Can you work these out from the model? Positions are in its coordinate system, mm. A direction names the side the tool comes from. Coordinates: 2 decimals unless noted, no trailing zeros. Order: outer loops, then holes, each group sorted by start corner. A loop starts at its lowest first (then second) coordinate and runs counter-clockwise, first axis right, second up.
```python
from build123d import *

# Parameters (mm, degrees)
SKETCH2_R           = 6
SKETCH2_R_2         = 1.5
BOSS_EXTRUDE1_DEPTH = 1.15
SKETCH3_R           = 4.4
BOSS_EXTRUDE2_DEPTH = 3.2
SKETCH4_R           = 0.75
BOSS_EXTRUDE3_DEPTH = 1.15
CIRPATTERN1_COUNT   = 2
CUT_EXTRUDE1_DEPTH  = 10


with BuildPart() as part:
    # Sketch2 → Boss-Extrude1 (new, symmetric)
    with BuildSketch(Plane(origin=(0, 0, 0), x_dir=(1, 0, 0), z_dir=(0, 1, 0))):
        with Locations(Location((0, 0, 0), (0, 0, 270))):
            Circle(SKETCH2_R)
        with Locations(Location((0, 0, 0), (0, 0, 270))):
            Circle(SKETCH2_R_2, mode=Mode.SUBTRACT)
    extrude(amount=BOSS_EXTRUDE1_DEPTH, both=True)

    # Sketch3 → Boss-Extrude2 (add)
    with BuildSketch(Plane(origin=(0, 1.15, 0), x_dir=(1, 0, 0), z_dir=(0, 1, 0))):
        with Locations(Location((0, 0, 0), (0, 0, 270))):
            Circle(SKETCH3_R)
        with BuildLine():
            Line((0.107421435, 2.898009771), (0.338399731, 2.678709694))
            Line((0.338399731, 2.678709694), (0.61665913, 2.83367809))
            ThreePointArc((0.61665913, 2.83367809), (0.721200673, 2.808891167), (0.824752316, 2.780248841))
            Line((0.824752316, 2.780248841), (0.993936292, 2.510396512))
            Line((0.993936292, 2.510396512), (1.301992734, 2.591295993))
            ThreePointArc((1.301992734, 2.591295993), (1.397085655, 2.541289372), (1.490260976, 2.48779465))
            Line((1.490260976, 2.48779465), (1.587020181, 2.184345885))
            Line((1.587020181, 2.184345885), (1.905517346, 2.186093238))
            ThreePointArc((1.905517346, 2.186093238), (1.985186607, 2.11400902), (2.062131058, 2.039023173))
            Line((2.062131058, 2.039023173), (2.080385755, 1.721044772))
            Line((2.080385755, 1.721044772), (2.389311295, 1.643530205))
            ThreePointArc((2.389311295, 1.643530205), (2.448550984, 1.553897705), (2.504429862, 1.46213237))
            Line((2.504429862, 1.46213237), (2.443033042, 1.149604087))
            Line((2.443033042, 1.149604087), (2.722976028, 0.997698125))
            ThreePointArc((2.722976028, 0.997698125), (2.758063897, 0.896149284), (2.789366126, 0.793370413))
            Line((2.789366126, 0.793370413), (2.652175577, 0.505929549))
            Line((2.652175577, 0.505929549), (2.885546163, 0.289177003))
            ThreePointArc((2.885546163, 0.289177003), (2.894277512, 0.182092507), (2.899036259, 0.074758075))
            Line((2.899036259, 0.074758075), (2.694672167, -0.169534403))
            Line((2.694672167, -0.169534403), (2.866806821, -0.437514174))
            ThreePointArc((2.866806821, -0.437514174), (2.848633027, -0.543405812), (2.826549281, -0.648551587))
            Line((2.826549281, -0.648551587), (2.567852594, -0.834345885))
            Line((2.567852594, -0.834345885), (2.667935462, -1.136714727))
            ThreePointArc((2.667935462, -1.136714727), (2.623998452, -1.234759946), (2.576459817, -1.331110368))
            Line((2.576459817, -1.331110368), (2.279685399, -1.446732346))
            Line((2.279685399, -1.446732346), (2.301427906, -1.764491312))
            ThreePointArc((2.301427906, -1.764491312), (2.234488404, -1.84852957), (2.164481907, -1.930030589))
            Line((2.164481907, -1.930030589), (1.848277186, -1.968215294))
            Line((1.848277186, -1.968215294), (1.790313171, -2.281398419))
            ThreePointArc((1.790313171, -2.281398419), (1.704577232, -2.346149284), (1.616501638, -2.40767989))
            Line((1.616501638, -2.40767989), (1.30073492, -2.366028036))
            Line((1.30073492, -2.366028036), (1.166706475, -2.654956874))
            ThreePointArc((1.166706475, -2.654956874), (1.067561203, -2.696351809), (0.966950626, -2.734045809))
            Line((0.966950626, -2.734045809), (0.671462695, -2.615174535))
            Line((0.671462695, -2.615174535), (0.469791321, -2.861694623))
            ThreePointArc((0.469791321, -2.861694623), (0.363466377, -2.877132634), (0.25664255, -2.888621575))
            Line((0.25664255, -2.888621575), (0, -2.7))
            Line((0, -2.7), (-0.25664255, -2.888621575))
            ThreePointArc((-0.25664255, -2.888621575), (-0.363466377, -2.877132634), (-0.469791321, -2.861694623))
            Line((-0.469791321, -2.861694623), (-0.671462695, -2.615174535))
            Line((-0.671462695, -2.615174535), (-0.966950626, -2.734045809))
            ThreePointArc((-0.966950626, -2.734045809), (-1.067561203, -2.696351809), (-1.166706475, -2.654956874))
            Line((-1.166706475, -2.654956874), (-1.30073492, -2.366028036))
            Line((-1.30073492, -2.366028036), (-1.616501638, -2.40767989))
            ThreePointArc((-1.616501638, -2.40767989), (-1.704577232, -2.346149284), (-1.790313171, -2.281398419))
            Line((-1.790313171, -2.281398419), (-1.848277186, -1.968215294))
            Line((-1.848277186, -1.968215294), (-2.164481907, -1.930030589))
            ThreePointArc((-2.164481907, -1.930030589), (-2.234488404, -1.84852957), (-2.301427906, -1.764491312))
            Line((-2.301427906, -1.764491312), (-2.279685399, -1.446732346))
            Line((-2.279685399, -1.446732346), (-2.576459817, -1.331110368))
            ThreePointArc((-2.576459817, -1.331110368), (-2.623998452, -1.234759946), (-2.667935462, -1.136714727))
            Line((-2.667935462, -1.136714727), (-2.567852594, -0.834345885))
            Line((-2.567852594, -0.834345885), (-2.826549281, -0.648551587))
            ThreePointArc((-2.826549281, -0.648551587), (-2.848633027, -0.543405812), (-2.866806821, -0.437514174))
            Line((-2.866806821, -0.437514174), (-2.694672167, -0.169534403))
            Line((-2.694672167, -0.169534403), (-2.899036259, 0.074758075))
            ThreePointArc((-2.899036259, 0.074758075), (-2.894277512, 0.182092507), (-2.885546163, 0.289177003))
            Line((-2.885546163, 0.289177003), (-2.652175577, 0.505929549))
            Line((-2.652175577, 0.505929549), (-2.789366126, 0.793370413))
            ThreePointArc((-2.789366126, 0.793370413), (-2.758063897, 0.896149284), (-2.722976028, 0.997698125))
            Line((-2.722976028, 0.997698125), (-2.443033042, 1.149604087))
            Line((-2.443033042, 1.149604087), (-2.504429862, 1.46213237))
            ThreePointArc((-2.504429862, 1.46213237), (-2.448550984, 1.553897705), (-2.389311295, 1.643530205))
            Line((-2.389311295, 1.643530205), (-2.080385755, 1.721044772))
            Line((-2.080385755, 1.721044772), (-2.062131058, 2.039023173))
            ThreePointArc((-2.062131058, 2.039023173), (-1.985186607, 2.11400902), (-1.905517346, 2.186093238))
            Line((-1.905517346, 2.186093238), (-1.587020181, 2.184345885))
            Line((-1.587020181, 2.184345885), (-1.490260976, 2.48779465))
            ThreePointArc((-1.490260976, 2.48779465), (-1.397085655, 2.541289372), (-1.301992734, 2.591295993))
            Line((-1.301992734, 2.591295993), (-0.993936292, 2.510396512))
            Line((-0.993936292, 2.510396512), (-0.824752316, 2.780248841))
            ThreePointArc((-0.824752316, 2.780248841), (-0.721200673, 2.808891167), (-0.61665913, 2.83367809))
            Line((-0.61665913, 2.83367809), (-0.338399731, 2.678709694))
            Line((-0.338399731, 2.678709694), (-0.107421435, 2.898009771))
            ThreePointArc((-0.107421435, 2.898009771), (0, 2.9), (0.107421435, 2.898009771))
        make_face(mode=Mode.SUBTRACT)
    extrude(amount=BOSS_EXTRUDE2_DEPTH)

    # Sketch4 → Boss-Extrude3 (add, symmetric)
    with BuildSketch(Plane(origin=(0, 0, 0), x_dir=(1, 0, 0), z_dir=(0, 1, 0))):
        with BuildLine():
            Line((3.968626967, 4.5), (16.888114198, 2.469689731))
            ThreePointArc((16.888114198, 2.469689731), (19, 0), (16.888114198, -2.469689731))
            Line((16.888114198, -2.469689731), (3.968626967, -4.5))
            ThreePointArc((3.968626967, -4.5), (6, 0), (3.968626967, 4.5))
        make_face()
        with Locations(Location((16, 0, 0), (0, 0, 270))):
            Circle(SKETCH4_R, mode=Mode.SUBTRACT)
        with Locations(Location((13, 0, 0), (0, 0, 270))):
            Circle(SKETCH4_R, mode=Mode.SUBTRACT)
        with Locations(Location((10, 0, 0), (0, 0, 270))):
            Circle(SKETCH4_R, mode=Mode.SUBTRACT)
        with Locations(Location((7, 0, 0), (0, 0, 270))):
            Circle(SKETCH4_R, mode=Mode.SUBTRACT)
    boss_extrude3 = extrude(amount=BOSS_EXTRUDE3_DEPTH, both=True)

    # CirPattern1: Boss-Extrude3 ×2 about axis
    cirpattern1_axis = Axis((0, 0, 0), (0, 1, 0))
    for i in range(1, CIRPATTERN1_COUNT):
        add(boss_extrude3.rotate(cirpattern1_axis, i * 360 / CIRPATTERN1_COUNT))

    # Sketch6 → Cut-Extrude1 (cut)
    with BuildSketch(Plane.XZ.offset(1.15)):
        Polygon((-12.25, 0), (-12.25, 5.932687926), (-21.293207436, 5.932687926), (-21.293207436, 0), (-21.293207436, -7.371619722), (-12.25, -7.371619722), align=None)
    extrude(amount=-CUT_EXTRUDE1_DEPTH, mode=Mode.SUBTRACT)


solid = part.part
```
1. Imagine slicing it at D-D on x = 16. Please give me the cut outline in (y, z), then the cut area to 3 significant figures.
Completed:
outline: (-1.15, -2.61) - (1.15, -2.61) - (1.15, -0.75) - (-1.15, -0.75) - close; (-1.15, 0.75) - (1.15, 0.75) - (1.15, 2.61) - (-1.15, 2.61) - close
area: 8.55 mm2
2. On a 3-axis mill with a long thin cutter (end or side, diameter ignored), from which of +Z, -Z, +X, -X, +Y, -Y can I reach the whole of each face in a straight line? I mean faces 1 (the flat face through (1.3, 1.15, 1.2)), 2 (the flat face through (-8.17, 0.02, -3.84)). Say none if no direction works.
Completed:
face 1: +Y
face 2: -Z, -X, +Y, -Y
3. I'm going to push flat-ended pins straight in: pin 1 (4 mm diameter, centred on x = 0, z = 0, fed in from +Y); pin 2 (1.5 mm diameter, centred on x = 6, y = -0.5, fed in from -Z). Where does each tip first touch, or does it pass through?
Completed:
pin 1: stops at y = 1.15
pin 2: stops at z = -4.3
4. Please list where these lines run through material, in increasing order: probe 1 along Y at (x, z) = (-9.5, -1.5); probe 2 along Z at (x, y) = (-7, 0.2); probe 3 along Z at (x, y) = (-6.5, -0.2).
Completed:
probe 1: y = -1.15 to 1.15
probe 2: z = -4.02 to -0.75, 0.75 to 4.02
probe 3: z = -4.1 to -0.56, 0.56 to 4.1
5. Imagine slicing it at A-A on x = 7. Please give me the cut outline in (y, z), then the cut area to 3 significant figures.
Completed:
outline: (-1.15, -4.02) - (1.15, -4.02) - (1.15, -0.75) - (-1.15, -0.75) - close; (-1.15, 0.75) - (1.15, 0.75) - (1.15, 4.02) - (-1.15, 4.02) - close
area: 15.1 mm2
6. Thinking about a two-plate mould opening in X: for faces 3 (the flat face through (4, 1.15, 3)), 4 (the flat face through (10.52, 0.02, 3.47)), 5 (the cylindrical face through (0.45, -0.02, 1.43)), 6 (the cylindrical face through (10.632, -0.016, 0.403)), which applies, pulls with the +X half, pulls with the -X half, needs draft (parallel to the pull), parting line crosses it, or undercut?
Completed:
face 3: needs draft
face 4: pulls with the +X half
face 5: undercut
face 6: undercut
7. Imagine slicing it at B-B on y = -0.25. Please give me the cut outline in (x, z).
Completed:
outline: (-12.25, -3.2) - (-3.97, -4.5) arc R6 ccw to (3.97, -4.5) - (16.89, -2.47) arc R2.5 ccw to (16.89, 2.47) - (3.97, 4.5) arc R6 ccw to (-3.97, 4.5) - (-12.25, 3.2) - close; hole circle Ø1.5 at (-10, 0); hole circle Ø1.5 at (-7, 0); hole circle Ø3 at (0, 0); hole circle Ø1.5 at (7, 0); hole circle Ø1.5 at (10, 0); hole circle Ø1.5 at (13, 0); hole circle Ø1.5 at (16, 0)
8. Imagine slicing it at C-C on z = 3.75. Please give me the cut outline in (x, y).
Completed:
outline: (-8.74, -1.15) - (8.74, -1.15) - (8.74, 1.15) - (2.3, 1.15) - (2.3, 4.35) - (-2.3, 4.35) - (-2.3, 1.15) - (-8.74, 1.15) - close
